Part model, mm, in its own coordinate system. A direction names the side the tool comes from. Give positions to 0.01 mm unless a question says otherwise; leave off trailing zeros. Order: outer loops, then holes, each group sorted by start corner. A loop starts at its lowest first (then second) coordinate and runs counter-clockwise, first axis right, second up. Notation, with made-up numbers: (89.5, -12) - (128.5, -12) arc R28 cw to (128.5, 25) - close; hole circle Ø11 at (1.25, -10). An arc over 180 degrees is marked (long way). One line per item, written item: value.
```python
from build123d import *

# Parameters (mm, degrees)
BOSS_EXTRUDE1_DEPTH = 5
SKETCH4_R           = 1.65
CUT_EXTRUDE1_DEPTH  = 5


with BuildPart() as part:
    # Sketch1 → Boss-Extrude1 (new body)
    with BuildSketch(Plane(origin=(0, 0, 0), x_dir=(0, 0, -1), z_dir=(1, 0, 0))):
        with BuildLine():
            Line((-44.040507459, 114.890413128), (-44.040507459, -43.329586872))
            Line((-44.040507459, -43.329586872), (-4.040507459, -43.329586872))
            Line((-4.040507459, -43.329586872), (96.679252091, 2.847191371))
            ThreePointArc((96.679252091, 2.847191371), (101.778005077, 7.275167621), (103.678182397, 13.755413128))
            Line((103.678182397, 13.755413128), (103.678182397, 57.805413128))
            ThreePointArc((103.678182397, 57.805413128), (101.778005077, 64.285658635), (96.679252091, 68.713634886))
            Line((96.679252091, 68.713634886), (-4.040507459, 114.890413128))
            Line((-4.040507459, 114.890413128), (-44.040507459, 114.890413128))
        make_face()
    extrude(amount=BOSS_EXTRUDE1_DEPTH)

    # Sketch4 → Cut-Extrude1 (cut)
    with BuildSketch(Plane(origin=(5, 0, 0), x_dir=(0, 0, -1), z_dir=(1, 0, 0))):
        with Locations((61.684952492, -7.146090177)):
            Circle(SKETCH4_R)
        with Locations(Location((61.684952492, 78.706916433, 0), (0, 0, 180))):
            Circle(SKETCH4_R)
        with BuildLine():
            Line((99.647066235, 57.119488088), (99.647066235, 46.419488088))
            ThreePointArc((99.647066235, 46.419488088), (97.997066235, 44.769488088), (96.347066235, 46.419488088))
            Line((96.347066235, 46.419488088), (96.347066235, 57.119488088))
            ThreePointArc((96.347066235, 57.119488088), (97.997066235, 58.769488088), (99.647066235, 57.119488088))
        make_face()
        with BuildLine():
            Line((99.647066235, 30.419488088), (99.647066235, 19.719488088))
            ThreePointArc((99.647066235, 19.719488088), (97.997066235, 18.069488088), (96.347066235, 19.719488088))
            Line((96.347066235, 19.719488088), (96.347066235, 30.419488088))
            ThreePointArc((96.347066235, 30.419488088), (97.997066235, 32.069488088), (99.647066235, 30.419488088))
        make_face()
        with BuildLine():
            Line((70.955654901, -0.999824899), (77.299153047, 1.959910101))
            ThreePointArc((77.299153047, 1.959910101), (79.492058003, 1.162308788), (78.69445669, -1.030596168))
            Line((78.69445669, -1.030596168), (72.350958543, -3.990331168))
            ThreePointArc((72.350958543, -3.990331168), (70.158053588, -3.192729855), (70.955654901, -0.999824899))
        make_face()
        with BuildLine():
            Line((70.955654901, 72.560651156), (77.299153047, 69.600916156))
            ThreePointArc((77.299153047, 69.600916156), (79.492058003, 70.398517469), (78.69445669, 72.591422424))
            Line((78.69445669, 72.591422424), (72.350958543, 75.551157424))
            ThreePointArc((72.350958543, 75.551157424), (70.158053588, 74.753556111), (70.955654901, 72.560651156))
        make_face()
    extrude(amount=-CUT_EXTRUDE1_DEPTH, mode=Mode.SUBTRACT)


solid = part.part
```
1) Cut at A-A, the plane y = 51. Give the cut face in (x, z), then the cut area to 3 significant figures.
Outcome:
outline: (0, -103.68) - (5, -103.68) - (5, -99.65) - (0, -99.65) - close; (0, -96.35) - (5, -96.35) - (5, 44.04) - (0, 44.04) - close
area: 722 mm^2
2) Cut at B-B, the plane x = 3. Give the cut face in (y, z).
Outcome:
outline: (-43.33, 4.04) - (2.85, -96.68) arc R12 ccw to (13.76, -103.68) - (57.81, -103.68) arc R12 ccw to (68.71, -96.68) - (114.89, 4.04) - (114.89, 44.04) - (-43.33, 44.04) - close; hole circle Ø3.3 at (-7.15, -61.68); hole (-3.99, -72.35) - (-1.03, -78.69) arc R1.65 ccw to (1.96, -77.3) - (-1, -70.96) arc R1.65 ccw to start; hole (19.72, -99.65) - (30.42, -99.65) arc R1.65 ccw to (30.42, -96.35) - (19.72, -96.35) arc R1.65 ccw to start; hole (46.42, -99.65) - (57.12, -99.65) arc R1.65 ccw to (57.12, -96.35) - (46.42, -96.35) arc R1.65 ccw to start; hole (69.6, -77.3) arc R1.65 ccw to (72.59, -78.69) - (75.55, -72.35) arc R1.65 ccw to (72.56, -70.96) - close; hole circle Ø3.3 at (78.71, -61.68)
3) Which spindle directions (+Z, -Z, +X, -X, +Y, -Y) get a long thin tool onto all of the face, cutting with end or side? Do faces 4 (the flat face through (2, 37, 44.041)), 5 (the flat face through (3, 52, -99.647)). Say none if no direction does.
Outcome:
face 4: +Z, +X, -X, +Y, -Y
face 5: +X, -X
4) Pin check, flat tips, straight feed: pin 1 (5.5 mm diameter, centred on y = 78.71, z = -61.68, fed in from +X); pin 2 (1.5 mm diameter, centred on x = 1.5, z = -38, fed in from -Y). Stop position of each tip, or through.
Outcome:
pin 1: stops at x = 5
pin 2: stops at y = -24.4
5) Cut at D-D, the plane y = 103. Give the cut face in (x, z), then the cut area to 3 significant figures.
Outcome:
outline: (0, -21.89) - (5, -21.89) - (5, 44.04) - (0, 44.04) - close
area: 330 mm^2
6) Cut at C-C, the plane z = -1. Give the cut face in (x, y).
Outcome:
outline: (0, -41.02) - (5, -41.02) - (5, 112.58) - (0, 112.58) - close
7) Drill centre lines: line 1 along Z through (x, y) = (4.7, 48.5); line 2 along Z through (x, y) = (4.2, -19); line 3 along Y through (x, z) = (1.4, -87). Where is each one in solid material? Low to high. Write a range as from..to.
Outcome:
line 1: z = -103.68..-99.65, -96.35..44.04
line 2: z = -49.03..44.04
line 3: y = -1.59..73.15
8) Mould opens along Z. For faces 1 (the flat face through (2.54, 74.05, -75.57)), 2 (the cylindrical face through (2.465, 7.195, -101.726)), 3 (the flat face through (2, -43.33, 24)) say: released by +Z, released by -Z, zero draft, split by the parting line, or undercut.
Outcome:
face 1: undercut
face 2: released by -Z
face 3: zero draft
